from build123d import *

# Parameters (mm, degrees)
SKETCH1_W               = 42
SKETCH1_H               = 32
PCB_DEPTH               = 1.6
MOUNT_HOLE_1_DEPTH      = 53.825751296
MOUNT_HOLE_1_DEPTH_BACK = 53.825751296
SKETCH2_R               = 1.5
MOUNT_HOLE_2_DEPTH      = 53.825751296
MOUNT_HOLE_2_DEPTH_BACK = 53.825751296
SKETCH3_R               = 1.5
MOUNT_HOLE_3_DEPTH      = 53.825751296
MOUNT_HOLE_3_DEPTH_BACK = 53.825751296
SKETCH4_R               = 1.5
MOUNT_HOLE_4_DEPTH      = 53.825751296
MOUNT_HOLE_4_DEPTH_BACK = 53.825751296
SKETCH5_R               = 1.5
BNC_SOCKET_START        = 1.6
SKETCH6_W               = 15
SKETCH6_H               = 12
BNC_SOCKET_DEPTH        = 12
OFFSET_POT_START        = 1.6
SKETCH7_W               = 9.5
SKETCH7_H               = 9.5
OFFSET_POT_DEPTH        = 10
LIMIT_POT_START         = 1.6
SKETCH8_W               = 9.5
SKETCH8_H               = 9.5
LIMIT_POT_DEPTH         = 10
OP_AMP_START            = 1.6
SKETCH9_W               = 5
SKETCH9_H               = 4
OP_AMP_DEPTH            = 1.5
HEADER_6PIN_START       = 1.6
SKETCH10_W              = 2.5
SKETCH10_H              = 15.2
HEADER_6PIN_DEPTH       = 8.5


with BuildPart() as part:
    # Sketch1 → PCB (new body)
    with BuildSketch(Plane(origin=(0, 0, 0), x_dir=(1, 0, 0), z_dir=(0, 1, 0))):
        with Locations((21, 16)):
            Rectangle(SKETCH1_W, SKETCH1_H)
    extrude(amount=PCB_DEPTH)

    # Sketch2 → Mount_hole_1 (cut, two sides: drawn at the far end of the back side and taken through both)
    with BuildSketch(Plane(origin=(0, 0, 0), x_dir=(1, 0, 0), z_dir=(0, 1, 0)).offset(-MOUNT_HOLE_1_DEPTH_BACK)):
        with Locations(Location((3, 3, 0), (0, 0, 270))):
            Circle(SKETCH2_R)
    extrude(amount=MOUNT_HOLE_1_DEPTH + MOUNT_HOLE_1_DEPTH_BACK, mode=Mode.SUBTRACT)

    # Sketch3 → Mount_hole_2 (cut, two sides: drawn at the far end of the back side and taken through both)
    with BuildSketch(Plane(origin=(0, 0, 0), x_dir=(1, 0, 0), z_dir=(0, 1, 0)).offset(-MOUNT_HOLE_2_DEPTH_BACK)):
        with Locations(Location((39, 3, 0), (0, 0, 270))):
            Circle(SKETCH3_R)
    extrude(amount=MOUNT_HOLE_2_DEPTH + MOUNT_HOLE_2_DEPTH_BACK, mode=Mode.SUBTRACT)

    # Sketch4 → Mount_hole_3 (cut, two sides: drawn at the far end of the back side and taken through both)
    with BuildSketch(Plane(origin=(0, 0, 0), x_dir=(1, 0, 0), z_dir=(0, 1, 0)).offset(-MOUNT_HOLE_3_DEPTH_BACK)):
        with Locations(Location((3, 29, 0), (0, 0, 270))):
            Circle(SKETCH4_R)
    extrude(amount=MOUNT_HOLE_3_DEPTH + MOUNT_HOLE_3_DEPTH_BACK, mode=Mode.SUBTRACT)

    # Sketch5 → Mount_hole_4 (cut, two sides: drawn at the far end of the back side and taken through both)
    with BuildSketch(Plane(origin=(0, 0, 0), x_dir=(1, 0, 0), z_dir=(0, 1, 0)).offset(-MOUNT_HOLE_4_DEPTH_BACK)):
        with Locations(Location((39, 29, 0), (0, 0, 270))):
            Circle(SKETCH5_R)
    extrude(amount=MOUNT_HOLE_4_DEPTH + MOUNT_HOLE_4_DEPTH_BACK, mode=Mode.SUBTRACT)

    # Sketch6 → BNC_socket (add)
    with BuildSketch(Plane(origin=(0, 0, 0), x_dir=(1, 0, 0), z_dir=(0, 1, 0)).offset(BNC_SOCKET_START)):
        with Locations((1.5, 16)):
            Rectangle(SKETCH6_W, SKETCH6_H)
    extrude(amount=BNC_SOCKET_DEPTH)

    # Sketch7 → Offset_pot (add)
    with BuildSketch(Plane(origin=(0, 0, 0), x_dir=(1, 0, 0), z_dir=(0, 1, 0)).offset(OFFSET_POT_START)):
        with Locations((22.75, 7.75)):
            Rectangle(SKETCH7_W, SKETCH7_H)
    extrude(amount=OFFSET_POT_DEPTH)

    # Sketch8 → Limit_pot (add)
    with BuildSketch(Plane(origin=(0, 0, 0), x_dir=(1, 0, 0), z_dir=(0, 1, 0)).offset(LIMIT_POT_START)):
        with Locations((22.75, 23.75)):
            Rectangle(SKETCH8_W, SKETCH8_H)
    extrude(amount=LIMIT_POT_DEPTH)

    # Sketch9 → Op_amp (add)
    with BuildSketch(Plane(origin=(0, 0, 0), x_dir=(1, 0, 0), z_dir=(0, 1, 0)).offset(OP_AMP_START)):
        with Locations((32.5, 15)):
            Rectangle(SKETCH9_W, SKETCH9_H)
    extrude(amount=OP_AMP_DEPTH)

    # Sketch10 → Header_6pin (add)
    with BuildSketch(Plane(origin=(0, 0, 0), x_dir=(1, 0, 0), z_dir=(0, 1, 0)).offset(HEADER_6PIN_START)):
        with Locations((40.25, 16)):
            Rectangle(SKETCH10_W, SKETCH10_H)
    extrude(amount=HEADER_6PIN_DEPTH)


solid = part.part
Could you check a few things on this model? Use its own coordinates, in mm. A direction names the side the tool comes from. Give positions to 0.01 mm unless a question says otherwise; leave off trailing zeros. Order: outer loops, then holes, each group sorted by start corner. A loop starts at its lowest first (then second) coordinate and runs counter-clockwise, first axis right, second up. Notation, with made-up numbers: (-14, 25.25) - (32, 25.25) arc R25 cw to (32, 61.25) - close; hole circle Ø2 at (82, 77.25). An arc over 180 degrees is marked (long way). Return JSON: item names as keys, results as strings. Group by question number.
Q1. Please list where these lines run through material, in increasing order: line 1 along Z through (x, y) = (3, 0.55); line 2 along X through (y, z) = (0.4, -29); line 3 along X through (y, z) = (6.5, -17.5). Write a range as [from, to].
Q2. Will these pins go through, and if not, where does the flat tip stop? pin 1 Ø5 at (x, y) = (1.5, 11) entering from -Z; pin 2 Ø16 at (x, z) = (22, -21) entering from +Y; pin 3 Ø4 at (x, y) = (12.5, 4) entering from -Z; pin 4 Ø7.5 at (y, z) = (6, -6) entering from +X.
Q3. Suppose I cut it at B-B, the plane z = -29. Please give me the cut outline in (x, y).
Q4. Thinking about a two-plate mould opening in Z: for faces 1 (the face through (23, 7, -19)), 2 (the face through (40, 6, -8.4)), 3 (the face through (42, 1, -16)), which applies, pulls with the +Z half, pulls with the -Z half, needs draft (parallel to the pull), parting line crosses it, or undercut?
Q5. Suppose I cut it at C-C, the plane y = 5. Please give me the cut outline in (x, z), and give its area (4 significant figures).
Q6. Suppose I cut it at D-D, the plane y = 11. Please give me the cut outline in (x, z), and give its area (4 significant figures).
Q7. Suppose I cut it at A-A, the plane x = 3. Please give me the cut outline in (y, z), and give its area (3 significant figures).
Q8. Which directions (+Z, -Z, +X, -X, +Y, -Y) give clear straight access to the entire face, cutting with the end or side of a thin tool? Please do faces 4 (the face through (41.5, 6, -16)), 5 (the face through (18, 7, -24)), 6 (the face through (0, 1, -16)).
Resolved:
{
 "1": {"line 1": "z = [-32, -30.5], [-27.5, -4.5], [-1.5, 0]", "line 2": "x = [0, 1.5], [4.5, 37.5], [40.5, 42]", "line 3": "x = [-6, 9], [39, 41.5]"},
 "2": {"pin 1": "stops at z = -22", "pin 2": "stops at y = 11.6", "pin 3": "passes through", "pin 4": "stops at x = 41.5"},
 "3": {"outline": "(0, 0) - (1.5, 0) - (1.5, 1.6) - (0, 1.6) - close; (4.5, 0) - (37.5, 0) - (37.5, 1.6) - (4.5, 1.6) - close; (40.5, 0) - (42, 0) - (42, 1.6) - (40.5, 1.6) - close"},
 "4": {"face 1": "undercut", "face 2": "pulls with the +Z half", "face 3": "needs draft"},
 "5": {"outline": "(-6, -22) - (9, -22) - (9, -10) - (-6, -10) - close; (18, -28.5) - (27.5, -28.5) - (27.5, -19) - (18, -19) - close; (18, -12.5) - (27.5, -12.5) - (27.5, -3) - (18, -3) - close; (39, -23.6) - (41.5, -23.6) - (41.5, -8.4) - (39, -8.4) - close", "area": "398.5 mm2"},
 "6": {"outline": "(-6, -22) - (9, -22) - (9, -10) - (-6, -10) - close; (18, -28.5) - (27.5, -28.5) - (27.5, -19) - (18, -19) - close; (18, -12.5) - (27.5, -12.5) - (27.5, -3) - (18, -3) - close", "area": "360.5 mm2"},
 "7": {"outline": "(0, -32) - (1.6, -32) - (1.6, -30.5) - (0, -30.5) - close; (0, -27.5) - (1.6, -27.5) - (1.6, -22) - (13.6, -22) - (13.6, -10) - (1.6, -10) - (1.6, -4.5) - (0, -4.5) - close; (0, -1.5) - (1.6, -1.5) - (1.6, 0) - (0, 0) - close", "area": "186 mm2"},
 "8": {"face 4": "+Z, -Z, +X, +Y", "face 5": "+Z, -Z, +Y", "face 6": "+Z, -Z, -X, -Y"}
}
